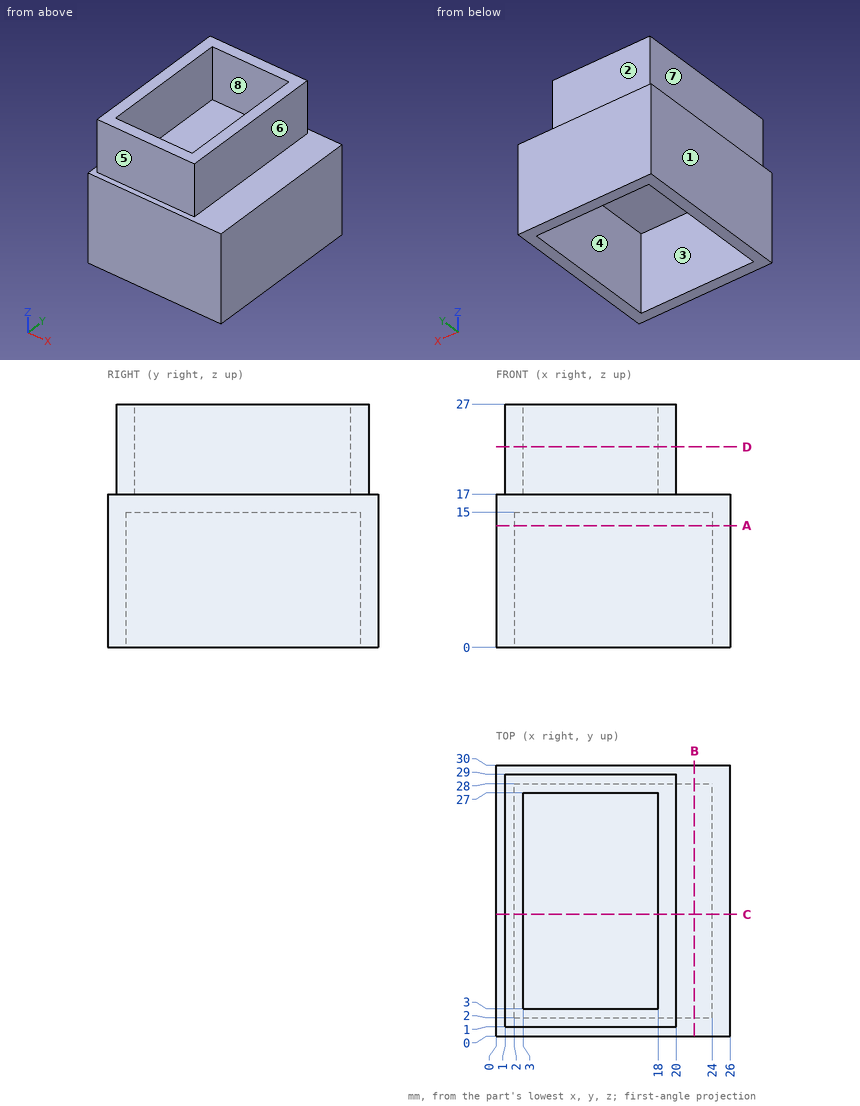
Input: dimensioned drawing with shaded views. Units: mm. Origin: part minimum x, y, z. A direction names the side the tool comes from. Coordinates: 2 decimals unless noted, no trailing zeros. Order: outer loops, then holes, each group sorted by start corner. A loop starts at its lowest first (then second) coordinate and runs counter-clockwise, first axis right, second up.
Item 1: Access query for the marked faces 4, 5, 6, 7 and 8. Directions: +Z, -Z, +X, -X, +Y, -Y. A direction counts if a zero-diameter tool reaches every point of the face in a straight line with its end or side. Return the directions, or none.
Answer:
face 4: -Z
face 5: +Z, +X, -X, -Y
face 6: +Z, +X, +Y, -Y
face 7: +Z, -X, +Y, -Y
face 8: +Z
Item 2: Section query B-B (x = 22). Output: boundary loops of the cut face in (y, z), then the cut area to 3 significant figures.
Answer:
outline: (0, 0) - (2, 0) - (2, 15) - (28, 15) - (28, 0) - (30, 0) - (30, 17) - (0, 17) - close
area: 120 mm2
Item 3: Material intervals for line 1 along X through (y, z) = (13.75, 4); line 2 along X through (y, z) = (19, 20); line 3 along Y through (x, z) = (13.75, 25.25), sorted ascending.
Answer:
line 1: x = 0 to 2, 24 to 26
line 2: x = 1 to 3, 18 to 20
line 3: y = 1 to 3, 27 to 29
Item 4: Contact query for flat-ended pins moving along their axis: P1, Ø6, axis at x = 14.5, y = 9, coming from the -Z side; P2, Ø5, axis at y = 11.5, z = 24, coming from the -X side; P3, Ø3, axis at y = 16, z = 20, coming from the +X side. Output: stop coordinate, or through.
Answer:
P1: stops at z = 15
P2: stops at x = 1
P3: stops at x = 20
Item 5: Section query C-C (y = 13.5). Output: boundary loops of the cut face in (x, z), then the cut area to 3 significant figures.
Answer:
outline: (0, 0) - (2, 0) - (2, 15) - (24, 15) - (24, 0) - (26, 0) - (26, 17) - (20, 17) - (20, 27) - (18, 27) - (18, 17) - (3, 17) - (3, 27) - (1, 27) - (1, 17) - (0, 17) - close
area: 152 mm2
Item 6: Section query A-A (z = 13.5). Output: boundary loops of the cut face in (x, y).
Answer:
outline: (0, 0) - (26, 0) - (26, 30) - (0, 30) - close; hole (2, 2) - (24, 2) - (24, 28) - (2, 28) - close
Item 7: Section query D-D (z = 22.25). Output: boundary loops of the cut face in (x, y), then the cut area to 3 significant figures.
Answer:
outline: (1, 1) - (20, 1) - (20, 29) - (1, 29) - close; hole (3, 3) - (18, 3) - (18, 27) - (3, 27) - close
area: 172 mm2
Item 8: Draft query along X for the marked faces 1, 2 and 3. Return one class per face: released by +X, released by -X, zero draft, split by the parting line, or undercut.
Answer:
face 1: released by -X
face 2: zero draft
face 3: undercut
